```python
from build123d import *

# Parameters (mm, degrees)
SKETCH1_R                = 33.3375
BOSS_EXTRUDE1_DEPTH      = 10
SKETCH2_R                = 1.5875
F_5_16_18_TAPPED_HOLE1_D = 6.5278


with BuildPart() as part:
    # Sketch1 → Boss-Extrude1 (new body)
    with BuildSketch(Plane(origin=(0, 0, 0), x_dir=(1, 0, 0), z_dir=(0, 1, 0))):
        Circle(SKETCH1_R)
    extrude(amount=BOSS_EXTRUDE1_DEPTH)

    # Sketch2 → Cut-Revolve1 (revolve, cut)
    with BuildSketch(Plane.XY):
        with Locations((33.3375, 5)):
            Circle(SKETCH2_R)
    revolve(axis=Axis((0, 10, 0), (0, -1, 0)), mode=Mode.SUBTRACT)

    # 5/16-18 Tapped Hole1 (through all)
    with Locations(Plane(origin=(0, 10, 0), x_dir=(1, 0, 0), z_dir=(0, 1, 0))):
        with Locations((0, 0)):
            Hole(F_5_16_18_TAPPED_HOLE1_D / 2)


solid = part.part
```
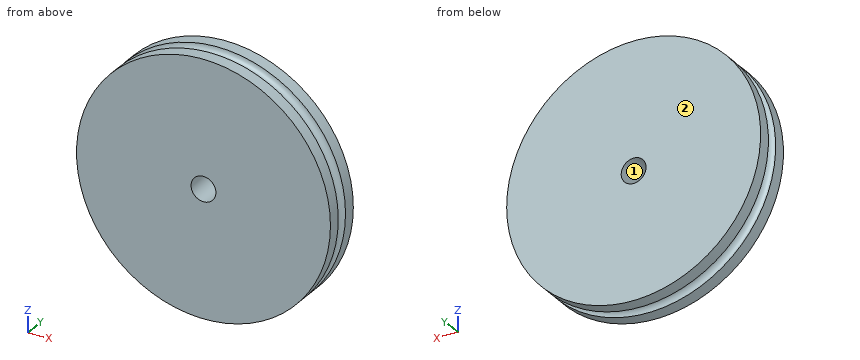
Geometry check sheet. Reference: the model listing, model coordinates, mm. Face numbers are marked on the shaded views. Coordinates: 2 decimals unless noted, no trailing zeros. Order: outer loops, then holes, each group sorted by start corner. A loop starts at its lowest first (then second) coordinate and runs counter-clockwise, first axis right, second up.
Item 1: Scan lines: line 1 along Z through (x, y) = (0, 7.75); line 2 along Y through (x, z) = (25.5, 21); line 3 along Z through (x, y) = (-1, 4.25). Record each from-to range of solid material in increasing order.
Item 2: Section check B-B (x = 0). Enter the section's corners in (y, z) (1 decimal), plus the area to 3 significant figures.
Item 3: Depth check by flat-ended pin: pin 1 (1 mm diameter, centred on y = 9, z = -12, fed in from -X); pin 2 (1 mm diameter, centred on y = 7, z = -7, fed in from -X); pin 3 (3 mm diameter, centred on y = 7, z = 24.5, fed in from -X); pin 4 (12 mm diameter, centred on x = -5.5, z = 10.5, fed in from -Y). Enter the tip coordinate at first touch or a pass-through.
Item 4: Mould release check, pull along X, two halves, no side actions. Record for the marked faces 1 and 2: released by +X, released by -X, zero draft, split by the parting line, or undercut.
Item 5: Section check D-D (y = 5.25). Enter the section's corners in (x, z).
Item 6: Section check C-C (y = 1.25). Enter the section's corners in (x, z) (1 decimal).
Item 7: Section check A-A (z = 0). Enter the section's corners in (x, y) (1 decimal).
Check sheet entries:
1. line 1: z = -33.34 to -3.26, 3.26 to 33.34
1. line 2: y = 0 to 3.44, 6.56 to 10
1. line 3: z = -31.92 to -3.11, 3.11 to 31.92
2. outline: (0, -33.3) - (3.4, -33.3) arc R1.6 cw to (6.6, -33.3) - (10, -33.3) - (10, -3.3) - (0, -3.3) - close; (0, 3.3) - (10, 3.3) - (10, 33.3) - (6.6, 33.3) arc R1.6 cw to (3.4, 33.3) - (0, 33.3) - close
2. area: 594 mm2
3. pin 1: stops at x = -31.29
3. pin 2: stops at x = -32.7
3. pin 3: stops at x = -24.13
3. pin 4: stops at y = 0
4. face 1: undercut
4. face 2: zero draft
5. outline: circle Ø63.54 at (0, 0); hole circle Ø6.53 at (0, 0)
6. outline: circle Ø66.7 at (0, 0); hole circle Ø6.5 at (0, 0)
7. outline: (-33.3, 0) - (-3.3, 0) - (-3.3, 10) - (-33.3, 10) - (-33.3, 6.6) arc R1.6 cw to (-33.3, 3.4) - close; (3.3, 0) - (33.3, 0) - (33.3, 3.4) arc R1.6 cw to (33.3, 6.6) - (33.3, 10) - (3.3, 10) - close
